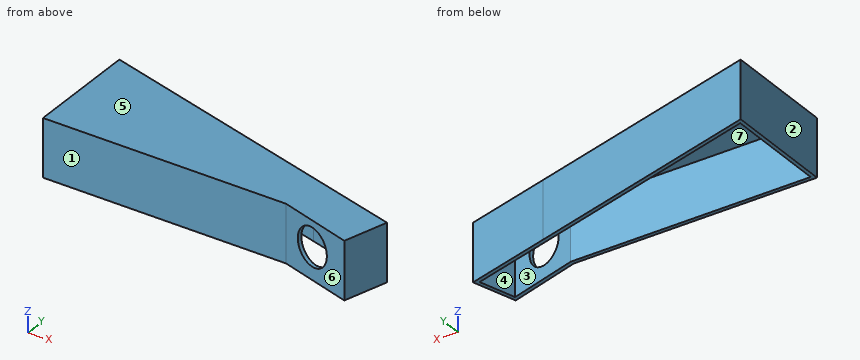
```python
from build123d import *

# Parameters (mm, degrees)
F1_DEPTH = 38
F2_T     = -2.5
F3_R     = 12.5
F4_DEPTH = 5


with BuildPart() as f1:
    # F0 (on Top) → F1 (new body)
    with BuildSketch(Plane.XY):
        Polygon((216.3945465859, -59.4591971258), (159.9115557721, -43.9392436979), (0, 0), (0, -73.9392436979), (159.9115557721, -73.9392436979), (207.8314225052, -88.2111171656), align=None)
    extrude(amount=F1_DEPTH)

    # F2
    f2_openings = [f1.faces().sort_by_distance(p)[0] for p in [
        (87.639416, -49.571978, 0),
    ]]
    offset(amount=F2_T, openings=f2_openings, kind=Kind.INTERSECTION)

    # F3 (on face) → F4 (cut)
    with BuildSketch(Plane(origin=(-7.1982832096, -24.1692706211, 0), x_dir=(0.9583973347, -0.2854374694, 0), z_dir=(-0.2854374694, -0.9583973347, 0))):
        with Locations((196.8638394408, 21)):
            Circle(F3_R)
    extrude(amount=-F4_DEPTH, mode=Mode.SUBTRACT)


solid = f1.part
```
Model file for the job. Use its own axes, mm. Face numbers are marked on the shaded views. A direction names the side the tool comes from. Give positions to 0.01 mm unless a question says otherwise; leave off trailing zeros. Order: outer loops, then holes, each group sorted by start corner. A loop starts at its lowest first (then second) coordinate and runs counter-clockwise, first axis right, second up.
1) Mould opens along Y. For the marked faces 4, 5, 6 and 7 say: +Y half, -Y half, draft (parallel to the pull), parting line (faces both ways), or undercut.
2) Wall check: probe 1 along Z at (x, y) = (125, -37.5); probe 2 along Y at (x, z) = (118.5, 15.5); probe 3 along Y at (x, z) = (116, 4). Give the ranges that are in metal, low to high.
3) Saw through at D-D, the plane z = 26.5. Write the cut outline in (x, y).
4) 3-axis set-ups, long thin cutter, end or side, ignore diameter. For the marked faces 1, 2 and 3: which of +Z, -Z, +X, -X, +Y, -Y reach the whole face in a straight line?
5) Saw through at B-B, the plane y = -57. Write the cut outline in (x, z).
6) Pin check, flat tips, straight feed: pin 1 (10.5 mm diameter, centred on x = 54.5, z = 22, fed in from +Y); pin 2 (11.5 mm diameter, centred on x = 63, z = 28, fed in from -Y); pin 3 (8 mm diameter, centred on x = 69, z = 27, fed in from +Y). Stop position of each tip, or through.
7) Saw through at C-C, the plane x = 143.5. Write the cut outline in (y, z).
8) Saw through at A-A, the plane z = 4. Write the cut outline in (x, y), then the cut area to 3 significant figures.
Computed:
1. face 4: undercut
1. face 5: draft
1. face 6: -Y half
1. face 7: undercut
2. probe 1: z = 35.5 to 38
2. probe 2: y = -73.94 to -71.44, -35.15 to -32.56
2. probe 3: y = -73.94 to -71.44, -34.47 to -31.87
3. outline: (0, -73.94) - (159.91, -73.94) - (170.72, -77.16) - (171.43, -74.76) - (160.28, -71.44) - (2.5, -71.44) - (2.5, -3.28) - (213.27, -61.19) - (206.15, -85.1) - (192.95, -81.17) - (192.23, -83.57) - (207.83, -88.21) - (216.39, -59.46) - (0, 0) - close
4. face 1: +Z, -Z, -X, -Y
4. face 2: +Z, -Z, -X, +Y, -Y
4. face 3: -Z
5. outline: (0, 0) - (2.5, 0) - (2.5, 35.5) - (198.01, 35.5) - (198.01, 0) - (207.44, 0) - (207.44, 38) - (0, 38) - close
6. pin 1: stops at y = -13.53
6. pin 2: stops at y = -73.94
6. pin 3: stops at y = -17.86
7. outline: (-73.94, 0) - (-71.44, 0) - (-71.44, 35.5) - (-42.02, 35.5) - (-42.02, 0) - (-39.43, 0) - (-39.43, 38) - (-73.94, 38) - close
8. outline: (0, -73.94) - (159.91, -73.94) - (207.83, -88.21) - (216.39, -59.46) - (0, 0) - close; hole (2.5, -71.44) - (160.28, -71.44) - (206.15, -85.1) - (213.27, -61.19) - (2.5, -3.28) - close
8. area: 1,320 mm2
